Read the model definition and answer for the solid it produces. Units are mm, in the model's axes. Face numbers are marked on the shaded views. A direction names the side the tool comes from. Give positions to 0.01 mm unless a question says otherwise; leave off trailing zeros. Write each loop counter-clockwise with the first axis right and the second up, starting at its lowest first coordinate (ties: lowest second). Pieces come first, ordered by that corner, then holes. Notation, with made-up numbers: (62, -27.75) -> (111, -27.75) arc R24 ccw to (111, 3.25) -> close; hole circle Ø10 at (29.25, 11). An arc over 180 degrees is marked (long way). Put each result on its own line as item: value. Start each with the question number.
from build123d import *

# Parameters (mm, degrees)
MAINBASESKETCH_W             = 31.8
MAINBASESKETCH_H             = 3.2
MAINBASEEXTRUDE_DEPTH        = 7.9
STUDSSKETCH_R                = 2.4
STUDSEXTRUDE_DEPTH           = 1.6
STUDSPATTERN_COUNT           = 2
STUDSPATTERN_PITCH           = 8
STUDSPATTERN_COUNT_DIR2      = 4
STUDSPATTERN_PITCH_DIR2      = 8
MAINBASESHELL_T              = -1.2
UNDERSIDECIRCLEEXT_START     = -0.2
UNDERSIDECIRCLESKETCH_R      = 3.14
UNDERSIDECIRCLESKETCH_R_2    = 2.4
UNDERSIDECIRCLEEXT_DEPTH     = 1.6
UNDERSIDECIRCLEPATTERN_COUNT = 3
UNDERSIDECIRCLEPATTERN_PITCH = 8


with BuildPart() as part:
    # MainBaseSketch → MainBaseExtrude (new, symmetric)
    with BuildSketch(Plane.XY):
        with Locations((16.581967213, 1.6)):
            Rectangle(MAINBASESKETCH_W, MAINBASESKETCH_H)
    extrude(amount=MAINBASEEXTRUDE_DEPTH, both=True)

    # StudsSketch → StudsExtrude (add)
    with BuildSketch(Plane(origin=(0, 3.2, 0), x_dir=(1, 0, 0), z_dir=(0, 1, 0))):
        with Locations((4.581967213, 4)):
            Circle(STUDSSKETCH_R)
    studsextrude = extrude(amount=STUDSEXTRUDE_DEPTH)

    # StudsPattern: StudsExtrude 2 × 4
    with Locations(*[(j * STUDSPATTERN_PITCH_DIR2, 0, i * STUDSPATTERN_PITCH) for i in range(STUDSPATTERN_COUNT) for j in range(STUDSPATTERN_COUNT_DIR2) if (i, j) != (0, 0)]):
        add(studsextrude)

    # MainBaseShell
    mainbaseshell_openings = [part.faces().sort_by_distance(p)[0] for p in [
        (16.581967213, 0, 0),
    ]]
    offset(amount=MAINBASESHELL_T, openings=mainbaseshell_openings, kind=Kind.INTERSECTION)

    # UnderSideCircleSketch → UnderSideCircleExt (add)
    with BuildSketch(Plane.XZ.offset(-2).offset(UNDERSIDECIRCLEEXT_START)):
        with Locations((8.581967213, 0)):
            Circle(UNDERSIDECIRCLESKETCH_R)
        with Locations((8.581967213, 0)):
            Circle(UNDERSIDECIRCLESKETCH_R_2, mode=Mode.SUBTRACT)
    undersidecircleext = extrude(amount=UNDERSIDECIRCLEEXT_DEPTH)

    # UnderSideCirclePattern: UnderSideCircleExt ×3
    with Locations(*[(i * UNDERSIDECIRCLEPATTERN_PITCH, 0, 0) for i in range(1, UNDERSIDECIRCLEPATTERN_COUNT)]):
        add(undersidecircleext)


solid = part.part
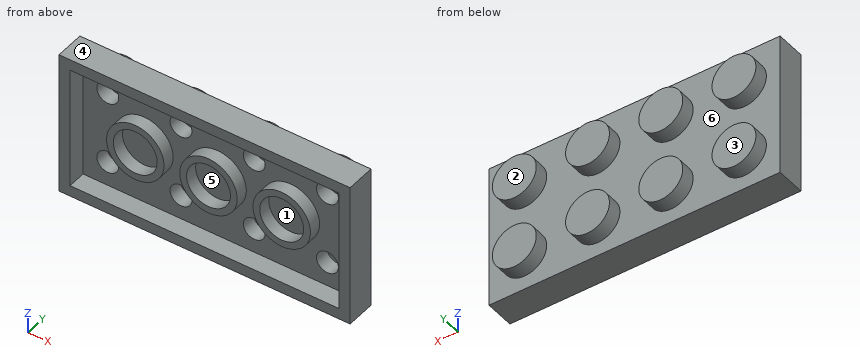
1) For the marked faces 1 and 2, determine the directions among +Z, -Z, +X, -X, +Y, -Y from which every point of the face is accessible in a straight line to the end or side of a thin tool.
2) Straight lines are drawn through the part: line 1 (Z direction, x = 28.5, y = 0.7); line 2 (X direction, y = 3.85, z = -2); line 3 (Y direction, x = 18, z = -1.25). For each, find the intervals that lie inside material, in ascending order. Write a range as [from, to].
3) A cutting plane is placed at C-C on x = 13. Give the vertices of the cut face in (y, z), and give its area (3 significant figures).
4) A cutting plane is placed at A-A on y = 2.45. State how many separate pieces and enclosed holes the cut face has, and give its area (3 significant figures).
5) Each of these flat-tipped pins is pushed along its axis until it touches: pin 1 Ø3 at (x, z) = (28.58, -4) entering from -Y; pin 2 Ø1.9 at (x, z) = (12.58, -4) entering from -Y; pin 3 Ø7 at (x, z) = (9, 0.5) entering from -Y. Where does it stop, or does it pass through?
6) For a pull along Z with two mould halves and no side action, classify the marked faces 3, 4, 5 and 6 as pulls with the +Z half, pulls with the -Z half, needs draft (parallel to the pull), parting line crosses it, or undercut.
Results found:
1. face 1: -Y
1. face 2: +Z, -Z, +X, -X, +Y
2. line 1: z = [-7.9, -6.7], [6.7, 7.9]
2. line 2: x = [3.26, 5.91], [11.26, 13.91], [19.26, 21.91], [27.26, 29.91]
2. line 3: y = [2, 3.2]
3. outline: (0, -7.9) -> (3.2, -7.9) -> (3.2, -6.36) -> (4.8, -6.36) -> (4.8, -1.64) -> (3.2, -1.64) -> (3.2, 1.64) -> (4.8, 1.64) -> (4.8, 6.36) -> (3.2, 6.36) -> (3.2, 7.9) -> (0, 7.9) -> (0, 6.7) -> (2, 6.7) -> (2, 5.12) -> (3.6, 5.12) -> (3.6, 2.88) -> (2, 2.88) -> (2, -2.88) -> (3.6, -2.88) -> (3.6, -5.12) -> (2, -5.12) -> (2, -6.7) -> (0, -6.7) -> close
3. area: 31.7 mm²
4. separate pieces: 1
4. enclosed holes: 8
4. area: 466 mm²
5. pin 1: stops at y = 2
5. pin 2: stops at y = 3.6
5. pin 3: stops at y = 0.6
6. face 3: needs draft
6. face 4: pulls with the +Z half
6. face 5: undercut
6. face 6: undercut
